CAD build for the part. Positions are in the model's coordinates, mm. A direction names the side the tool comes from. Coordinates: 2 decimals unless noted, no trailing zeros. Loops run counter-clockwise (first coordinate to the right, second up) from the corner with the lowest first, then second, coordinate; pieces in that order, holes last. Notation, with made-up numbers: (-4, 67.5) -> (32, 67.5) arc R18 ccw to (32, 78.5) -> close; hole circle Ø4 at (-30, 23.25). An arc over 180 degrees is marked (long way). Return JSON: item names as keys, results as strings. Group by question number.
(1) Saw through at C-C on y = 11.5. Write the cut outline in (x, z), then the cut area to 3 significant figures.
(2) Saw through at D-D on z = -4.5. Write the cut outline in (x, y), then the cut area to 3 significant figures.
(3) Saw through at A-A on z = 0. Write the cut outline in (x, y).
(4) Saw through at B-B on x = 0. Write the cut outline in (y, z), then the cut area to 4 significant figures.
(5) Tool access for faces 1 (the face through (-16, 1, 5.3)), 2 (the face through (-19, 10, 0)), 3 (the face through (0.208, 13.586, 18.695)), 4 (the face through (17.49, 8.34, 0.62)): list every direction of +Z, -Z, +X, -X, +Y, -Y with a clear straight run to the whole face (end or side of a thin tool).
(6) Probe L1, parallel to Y at x = 0, z = -17.95; L2, parallel to X at y = 6.25, z = 0; L3, parallel to X at y = 3.5, z = -12. List the from-to ranges inside material, lowest first.
(7) Flat gauge pins, fed straight in: pin 1 Ø5 at (y, z) = (12, -2) entering from -X; pin 2 Ø3 at (y, z) = (12, 0) entering from -X; pin 3 Ø4 at (x, y) = (-11, 5) entering from +Z; pin 4 Ø1 at (y, z) = (1.5, -2.5) entering from -X. Where does each tip first touch, or does it go through?
(8) Mould opens along Z. For faces 5 (the face through (0, 2, 0)), 6 (the face through (19.98, 7.15, -0.88)), 7 (the face through (18, 14.5, 0)) say: pulls with the +Z half, pulls with the -Z half, needs draft (parallel to the pull), parting line crosses it, or undercut.
Autodesk Inventor part; units mm, degrees
ref_plane "Work Plane1" through (20, 14.5, 0) normal (1, 0, 0) x (0, 1, 0)
ref_plane "Work Plane2" through (0, 14.5, -20) normal (0, 0, -1) x (-1, 0, 0)
ref_plane "YZ Plane" through (0, 0, 0) normal (1, 0, 0) x (0, 1, 0)
sketch "Sketch1" plane through (0, 0, 0) normal (0, 1, 0) x (-1, 0, 0)
  circle A0 centre (0, 0) radius 20
  dimension "d0" = 40
sketch "Sketch1 outline for Extrusion1" plane through (0, 0, 0) normal (0, 1, 0) x (-1, 0, 0)
  circle A0 centre (0, 0) radius 20
extrude "Extrusion1" add sketch "Sketch1 outline for Extrusion1" along normal blind 10
sketch "Sketch2" plane through (0, 10, 0) normal (0, 1, 0) x (1, 0, 0)
  circle A0 centre (0, 0) radius 17.5
  circle A1 centre (0, 0) radius 20
  line L0 (-18.330303, 8) -> (-15.564382, 8)
  line L1 (-18.330303, -8) -> (-15.564382, -8)
  circle A2 centre (0, 0) radius 20
  point P0 (-16.947343, 8)
  dimension "d3" = 35
  dimension "d4" = 8
  dimension "d5" = 8
  dimension "d6" = 40
sketch "Sketch2 outline for Extrusion2" plane through (0, 10, 0) normal (0, 1, 0) x (1, 0, 0)
  line L0 (-15.564382, -8) -> (-18.330303, -8)
  arc A0 (-15.564382, 8) -> (-15.564382, -8) centre (0, 0) cw
  line L1 (-18.330303, 8) -> (-15.564382, 8)
  arc A1 (-18.330303, -8) -> (-18.330303, 8) centre (0, 0) ccw
extrude "Extrusion2" add sketch "Sketch2 outline for Extrusion2" along normal blind 4.5
sketch "Sketch3" plane through (0, 10, 0) normal (0, 1, 0) x (1, 0, 0)
  circle A0 centre (0, 0) radius 17.5
sketch "Sketch3 outline for Extrusion3" plane through (0, 10, 0) normal (0, 1, 0) x (1, 0, 0)
  circle A0 centre (0, 0) radius 17.5
extrude "Extrusion3" cut sketch "Sketch3 outline for Extrusion3" against normal blind 8
sketch "Sketch4" plane through (0, 14.5, 0) normal (0, 1, 0) x (1, 0, 0)
  circle A0 centre (0, 0) radius 20
  point P0 (0, -20.035453)
  point P1 (20, 0)
  point P2 (0, 20)
ref_plane "Work Plane1" through (20, 14.5, 0) normal (1, 0, 0) x (0, 1, 0)
sketch "Sketch5" plane through (20, 14.5, 0) normal (1, 0, 0) x (0, 1, 0)
  circle A0 centre (-2.5, 0) radius 1.6
  line L0 (0, -20) -> (0, 20)
  point P0 (-14.5, 0)
  point P1 (0, 8)
  point P2 (0, -8)
  dimension "d11" = 3.2
  dimension "d12" = 2.5
sketch "Sketch5 outline for Extrusion4" plane through (20, 14.5, 0) normal (1, 0, 0) x (0, 1, 0)
  circle A0 centre (-2.5, 0) radius 1.6
extrude "Extrusion4" cut sketch "Sketch5 outline for Extrusion4" against normal up to surface
ref_plane "Work Plane2" through (0, 14.5, -20) normal (0, 0, -1) x (-1, 0, 0)
sketch "Sketch6" plane through (0, 14.5, -20) normal (0, 0, -1) x (-1, 0, 0)
  circle A0 centre (0, -2.5) radius 1.6
  line L0 (18.330303, 0) -> (-20, 0)
  point P0 (0, -14.5)
  dimension "d15" = 3.2
  dimension "d16" = 2.5
sketch "Sketch6 outline for Extrusion5" plane through (0, 14.5, -20) normal (0, 0, -1) x (-1, 0, 0)
  circle A0 centre (0, -2.5) radius 1.6
extrude "Extrusion5" cut sketch "Sketch6 outline for Extrusion5" against normal through all
sketch "Sketch7" plane through (0, 10, 0) normal (0, 1, 0) x (1, 0, 0)
  line L0 (-13, -3.3) -> (-13, 5.1)
  line L1 (-13, 5.1) -> (-18.25, 5.1)
  line L2 (-18.25, 5.1) -> (-18.25, -3.3)
  line L3 (-16.25, -5.3) -> (-15, -5.3)
  arc A0 (-15, -5.3) -> (-13, -3.3) centre (-15, -3.3) ccw
  arc A1 (-18.25, -3.3) -> (-16.25, -5.3) centre (-16.25, -3.3) ccw
  arc A2 (-18.330303, 8) -> (-18.330303, -8) centre (0, 0) ccw
  point P0 (-18.25, -5.3)
  dimension "d19" = 10.4
  dimension "d20" = 5.25
  dimension "d21" = 2
  dimension "d25" = 18.25
  dimension "d26" = 5.1
sketch "Sketch7 outline for Extrusion6" plane through (0, 10, 0) normal (0, 1, 0) x (1, 0, 0)
  line L0 (-13, -3.3) -> (-13, 5.1)
  arc A0 (-15, -5.3) -> (-13, -3.3) centre (-15, -3.3) ccw
  line L1 (-16.25, -5.3) -> (-15, -5.3)
  arc A1 (-18.25, -3.3) -> (-16.25, -5.3) centre (-16.25, -3.3) ccw
  line L2 (-18.25, 5.1) -> (-18.25, -3.3)
  line L3 (-13, 5.1) -> (-18.25, 5.1)
extrude "Extrusion6" cut sketch "Sketch7 outline for Extrusion6" against normal through all
properties part number "Payload Adapter"
Geometry results:
{
 "1": {"outline": "(-18.33, -8) arc R20 ccw to (-1.52, -19.94) -> (-1.52, -17.43) arc R17.5 cw to (-15.56, -8) -> close; (-18.33, 8) -> (-15.56, 8) arc R17.5 cw to (-1.52, 17.43) -> (-1.52, 19.94) arc R20 ccw to start; (1.52, -19.94) arc R20 ccw to (19.94, -1.52) -> (17.43, -1.52) arc R17.5 cw to (1.52, -17.43) -> close; (1.52, 17.43) arc R17.5 cw to (17.43, 1.52) -> (19.94, 1.52) arc R20 ccw to (1.52, 19.94) -> close", "area": "230 mm²"},
 "2": {"outline": "(-19.49, 0) -> (-18.25, 0) -> (-18.25, 10) -> (-19.49, 10) -> close; (-13, 0) -> (19.49, 0) -> (19.49, 14.5) -> (16.91, 14.5) -> (16.91, 2) -> (-13, 2) -> close", "area": "110 mm²"},
 "3": {"outline": "(-20, 0) -> (-18.25, 0) -> (-18.25, 10) -> (-20, 10) -> close; (-13, 0) -> (20, 0) -> (20, 10.4) -> (17.5, 10.4) -> (17.5, 2) -> (-13, 2) -> close; (17.5, 13.6) -> (20, 13.6) -> (20, 14.5) -> (17.5, 14.5) -> close"},
 "4": {"outline": "(0, -20) -> (10.4, -20) -> (10.4, -17.5) -> (2, -17.5) -> (2, 17.5) -> (10.4, 17.5) -> (10.4, 20) -> (0, 20) -> close; (13.6, -20) -> (14.5, -20) -> (14.5, -17.5) -> (13.6, -17.5) -> close; (13.6, 17.5) -> (14.5, 17.5) -> (14.5, 20) -> (13.6, 20) -> close", "area": "126.5 mm²"},
 "5": {"face 1": "+Y, -Y", "face 2": "-X, +Y", "face 3": "+Z, -Z", "face 4": "+Y"},
 "6": {"L1": "0 to 10.4, 13.6 to 14.5", "L2": "-20 to -18.25, 17.5 to 20", "L3": "-16 to -12.74, 12.74 to 16"},
 "7": {"pin 1": "x = -19.99", "pin 2": "through", "pin 3": "z = 17.86", "pin 4": "x = -19.9"},
 "8": {"face 5": "undercut", "face 6": "parting line crosses it", "face 7": "needs draft"}
}
